Read the model definition and answer for the solid it produces. Units are mm, in the model's axes. Coordinates: 2 decimals unless noted, no trailing zeros. Order: outer loops, then holes, each group sorted by start corner. A loop starts at its lowest first (then second) coordinate and runs counter-clockwise, first axis right, second up. Notation, with made-up numbers: (46.5, 6) -> (51.5, 6) arc R18 cw to (51.5, 34) -> close; hole circle Ø1 at (31.25, 32.5). An arc over 180 degrees is marked (long way). Use CSV: the item, a comma, the result in double quotes.
```python
from build123d import *

# Parameters (mm, degrees)
SKETCH1_R           = 11.43
SKETCH1_R_2         = 10.16
BOSS_EXTRUDE1_DEPTH = 46.99
BOSS_EXTRUDE2_START = 20
SKETCH3_R           = 1.85
SKETCH3_R_2         = 1.5
BOSS_EXTRUDE2_DEPTH = 2.5
CHAMFER4_SIZE       = 7.5
CHAMFER4_SIZE_2     = 4.330127019
CHAMFER5_SIZE       = 7.5
CHAMFER5_SIZE_2     = 4.330127019
SKETCH4_R           = 0.5
CUT_EXTRUDE1_DEPTH  = 5


with BuildPart() as part:
    # Sketch1 → Boss-Extrude1 (new body)
    with BuildSketch(Plane(origin=(0, 0, 0), x_dir=(1, 0, 0), z_dir=(0, 1, 0))):
        with Locations(Location((0, 0, 0), (0, 0, 270))):
            Circle(SKETCH1_R)
        with Locations(Location((0, 0, 0), (0, 0, 270))):
            Circle(SKETCH1_R_2, mode=Mode.SUBTRACT)
    extrude(amount=BOSS_EXTRUDE1_DEPTH)

    # Sketch3 → Boss-Extrude2 (add)
    with BuildSketch(Plane(origin=(0, 0, 0), x_dir=(1, 0, 0), z_dir=(0, 1, 0)).offset(BOSS_EXTRUDE2_START)):
        with Locations((13, 0)):
            Circle(SKETCH3_R)
        with Locations(Location((13, 0, 0), (0, 0, 270))):
            Circle(SKETCH3_R_2, mode=Mode.SUBTRACT)
    extrude(amount=BOSS_EXTRUDE2_DEPTH)

    # Chamfer4
    # the kernel refuses this chamfer: 7.5, 4.330127019 mm, written as the material it adds along each edge
    with BuildSketch(Plane(origin=(0, 20, 0), x_dir=(-0.2055966456613654, 0, -0.9786368168492308), z_dir=(-0.9786368168492308, 0, 0.2055966456613654))) as chamfer4_piece_1_section:
        Polygon((11.43, CHAMFER4_SIZE), (11.43 + CHAMFER4_SIZE_2, 0), (11.43, 0), align=None)
    chamfer4_piece_1 = revolve(axis=Axis((0, 20, 0), (0, -1, 0)), revolution_arc=203.728856682, mode=Mode.PRIVATE)
    chamfer4_piece_1 = chamfer4_piece_1 - Plane(origin=(13, 13.499486396, 0), x_dir=(0, 0, 1), z_dir=(0, -1, 0)) * Cylinder(1.5, 64, mode=Mode.PRIVATE)
    chamfer4_piece_1 = chamfer4_piece_1 & Plane(origin=(13, 13.499486396, 0), x_dir=(1, 0, 0), z_dir=(0, -1, 0)) * Cylinder(1.85, 64, mode=Mode.PRIVATE)
    add(chamfer4_piece_1)

    # Chamfer5
    # the kernel refuses this chamfer: 7.5, 4.330127019 mm, written as the material it adds along each edge
    with BuildSketch(Plane(origin=(0, 22.5, 0), x_dir=(-0.20559664566136496, 0, -0.9786368168492309), z_dir=(-0.9786368168492309, 0, 0.20559664566136496))) as chamfer5_piece_1_section:
        Polygon((11.43 + CHAMFER5_SIZE, 0), (11.43, -CHAMFER5_SIZE_2), (11.43, 0), align=None)
    chamfer5_piece_1 = revolve(axis=Axis((0, 22.5, 0), (0, -1, 0)), revolution_arc=203.728856682, mode=Mode.PRIVATE)
    chamfer5_piece_1 = chamfer5_piece_1 - Plane(origin=(13, 25.165434587, 0), x_dir=(0, 0, 1), z_dir=(0, -1, 0)) * Cylinder(1.5, 76, mode=Mode.PRIVATE)
    chamfer5_piece_1 = chamfer5_piece_1 & Plane(origin=(13, 25.165434587, 0), x_dir=(1, 0, 0), z_dir=(0, -1, 0)) * Cylinder(1.85, 76, mode=Mode.PRIVATE)
    add(chamfer5_piece_1)

    # Sketch4 → Cut-Extrude1 (cut)
    with BuildSketch(Plane(origin=(11.43, 0, 0), x_dir=(0, 0, -1), z_dir=(1, 0, 0))):
        with Locations((0, 30.132630437)):
            Circle(SKETCH4_R)
        with Locations((0, 32.632630437)):
            Circle(SKETCH4_R)
        with Locations((0, 35.132630437)):
            Circle(SKETCH4_R)
        with Locations((0, 37.632630437)):
            Circle(SKETCH4_R)
        with Locations((0, 40.132630437)):
            Circle(SKETCH4_R)
    extrude(amount=-CUT_EXTRUDE1_DEPTH, mode=Mode.SUBTRACT)


solid = part.part
```
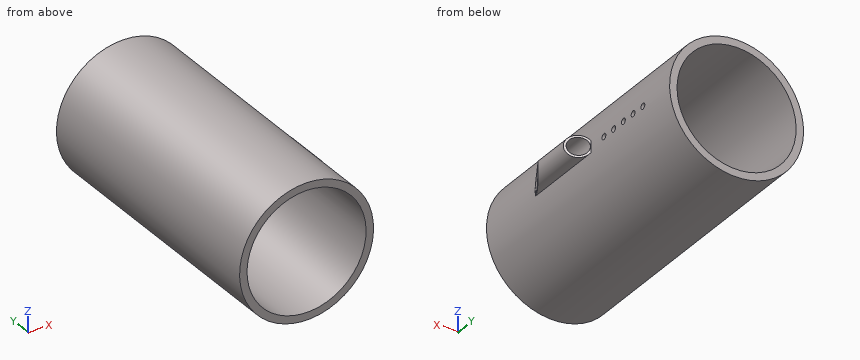
Item 1: Straight lines are drawn through the part: line 1 along Y through (x, z) = (11.1, 0); line 2 along X through (y, z) = (22.25, 0); line 3 along X through (y, z) = (14, -1.25). For each, find the intervals that lie inside material, in ascending order.
Return value:
line 1,"y = 0 to 29.63, 30.63 to 32.13, 33.13 to 34.63, 35.63 to 37.13, 38.13 to 39.63, 40.63 to 46.99"
line 2,"x = -11.43 to -10.16, 10.16 to 11.5, 14.5 to 14.85"
line 3,"x = -11.36 to -10.08, 10.08 to 11.36, 11.64 to 12.17"
Item 2: Find section D-D, the plane z = 0. Give the number of separate pieces and of enclosed holes in the cut face, then the cut area to 3 significant figures.
Return value:
separate pieces,"8"
enclosed holes,"0"
area,"116 mm^2"
Item 3: Find section B-B, the plane x = 0. Give the vertices of the cut face in (y, z), then the cut area to 3 significant figures.
Return value:
outline,"(0, -11.43) -> (46.99, -11.43) -> (46.99, -10.16) -> (0, -10.16) -> close; (0, 10.16) -> (46.99, 10.16) -> (46.99, 11.43) -> (0, 11.43) -> close"
area,"119 mm^2"
Item 4: Find section C-C, the plane y = 5.5. Give the vertices of the cut face in (x, z), then the cut area to 3 significant figures.
Return value:
outline,"circle Ø22.86 at (0, 0); hole circle Ø20.32 at (0, 0)"
area,"86.1 mm^2"
Item 5: Each of these flat-tipped pins is pushed along its axis until it touches: P1, Ø10, axis at y = 21.5, z = 7, coming from the -X side; P2, Ø8, axis at x = 7.5, y = 31.5, coming from the -Z side; P3, Ø3, axis at x = 7.5, y = 33.5, coming from the +Z side. Where does it stop, or does it pass through?
Return value:
P1,"stops at x = -11.25"
P2,"stops at z = -10.88"
P3,"stops at z = 9.73"
Item 6: Find section A-A, the plane z = 4. Give the vertices of the cut face in (x, y).
Return value:
outline,"(-10.71, 0) -> (-9.34, 0) -> (-9.34, 46.99) -> (-10.71, 46.99) -> close; (9.34, 0) -> (10.71, 0) -> (10.71, 46.99) -> (9.34, 46.99) -> close"
